CAD build for the part. Positions are in the model's coordinates, mm. A direction names the side the tool comes from. Round coordinates to 2 decimals unless told otherwise and drop trailing zeros. Loops run counter-clockwise (first coordinate to the right, second up) from the corner with the lowest first, then second, coordinate; pieces in that order, holes last.
Autodesk Fusion 360 part; units mm, degrees
box "BoxPrimitive1" add length 111 width 43 height 5 placed x (0, 1, 0) y (-1, 0, 0) z (0, 0, 1) at (43.0003, 0, 0)
sketch "Sketch6" plane through (0, 0, 0) normal (0, 0, -1) x (1, 0, 0)
  line L0 (0.0003, -111) -> (43.0003, -111)
  line L1 (43.0003, -111) -> (43.0003, 0)
  line L2 (43.0003, 0) -> (0.0003, 0)
  line L3 (0.0003, 0) -> (0.0003, -111)
  line L4 (0.0003, -93) -> (18.0003, -111)
  line L5 (6.5003, -22.25) -> (41.5003, -22.25) construction
  line L6 (41.5003, -22.25) -> (41.5003, -88.75) construction
  line L7 (41.5003, -88.75) -> (6.5003, -88.75) construction
  line L8 (6.5003, -88.75) -> (6.5003, -22.25) construction
  line L9 (6.5003, -22.25) -> (41.5003, -88.75) construction
  line L10 (6.5003, -88.75) -> (41.5003, -22.25) construction
  circle A0 centre (8.2003, -23.95) radius 0.8
  line L11 (38.2503, -87.75) -> (9.7503, -87.75)
  line L12 (9.7503, -87.75) -> (9.7503, -23.25)
  line L13 (9.7503, -23.25) -> (38.2503, -23.25)
  line L14 (38.2503, -23.25) -> (38.2503, -87.75)
  line L15 (38.2503, -87.75) -> (9.7503, -23.25) construction
  line L16 (9.7503, -87.75) -> (38.2503, -23.25) construction
  line L17 (18.2503, -91) -> (38.2503, -91)
  line L18 (38.2503, -91) -> (38.2503, -103)
  line L19 (38.2503, -103) -> (18.2503, -103)
  line L20 (18.2503, -103) -> (18.2503, -91)
  circle A1 centre (2.5003, -2.5) radius 1.2
  circle A2 centre (40.5003, -2.5) radius 1.2
  circle A3 centre (40.5003, -108.5) radius 1.2
  circle A4 centre (2.5003, -90.5) radius 1.2
  line L21 (24.0003, -111) -> (24.0003, 0) construction
  line L22 (0.0003, -55.5) -> (43.0003, -55.5) construction
  circle A5 centre (8.2003, -87.05) radius 0.8
  circle A6 centre (39.8003, -23.95) radius 0.8
  circle A7 centre (39.8003, -87.05) radius 0.8
  line L23 (18.2503, -91) -> (38.2503, -103) construction
  line L24 (38.2503, -91) -> (18.2503, -103) construction
  point P0 (24.0003, -55.5)
  point P1 (24.0003, -55.5)
  point P2 (24.0003, -55.5)
  point P3 (24.0003, -55.5)
  point P4 (28.2503, -97)
  dimension "d7" = 45
  dimension "d8" = 35
  dimension "d9" = 66.5
  dimension "d11" = 1.6
  dimension "d12" = 1.7
  dimension "d13" = 1.7
  dimension "d14" = 28.5
  dimension "d15" = 64.5
  dimension "d17" = 2.4
  dimension "d18" = 2.5
  dimension "d19" = 2.5
  dimension "d21" = 2.4
  dimension "d22" = 2.5
  dimension "d23" = 2.5
  dimension "d24" = 2.4
  dimension "d25" = 2.5
  dimension "d26" = 2.5
  dimension "d38" = 93
  dimension "d39" = 4.75
  dimension "d42" = 20
  dimension "d43" = 12
  dimension "d47" = 55.5
  dimension "d48" = 19
  dimension "d51" = 2.5
  dimension "d52" = 2.5
  dimension "d53" = 2.4
  dimension "d56" = 3.25
extrude "Extrude1" cut sketch "Sketch6" against normal through all contours L0 L3 L4 | L11 L12 L13 L14 | L17 L18 L19 L20 | A1 | A2 | A3 | A4
extrude "Extrude4" cut sketch "Sketch6" against normal blind 4 contours A0 | A5 | A6 | A7
thread "Thread2" thread offset 0 thread length 10
sketch "Sketch9" plane through (0, 0, 5) normal (0, 0, 1) x (-1, 0, 0)
  line L0 (-18.0003, -111) -> (-0.0003, -93)
  line L1 (-0.0003, -93) -> (-0.0003, 0)
  line L2 (-0.0003, 0) -> (-43.0003, 0)
  line L3 (-43.0003, 0) -> (-43.0003, -111)
  line L4 (-43.0003, -111) -> (-18.0003, -111)
  circle A0 centre (-40.5003, -108.5) radius 1.2
  line L5 (-18.2503, -91) -> (-18.2503, -103)
  line L6 (-18.2503, -103) -> (-38.2503, -103)
  line L7 (-38.2503, -103) -> (-38.2503, -91)
  line L8 (-38.2503, -91) -> (-18.2503, -91)
  circle A1 centre (-2.5003, -90.5) radius 1.2
  circle A2 centre (-40.5003, -2.5) radius 1.2
  line L9 (-38.2503, -87.75) -> (-38.2503, -23.25)
  line L10 (-38.2503, -23.25) -> (-9.7503, -23.25)
  line L11 (-9.7503, -23.25) -> (-9.7503, -87.75)
  line L12 (-9.7503, -87.75) -> (-38.2503, -87.75)
  circle A3 centre (-2.5003, -2.5) radius 1.2
  circle A4 centre (-2.5003, -2.5) radius 2
  circle A5 centre (-40.5003, -2.5) radius 2
  circle A6 centre (-2.5003, -90.5) radius 2
  circle A7 centre (-40.5003, -108.5) radius 2
  dimension "d32" = 4
  dimension "d33" = 4
  dimension "d34" = 4
  dimension "d35" = 4
extrude "Extrude3" cut sketch "Sketch9" against normal blind 2.5 contours A4 | A5 | A6 | A7
sketch "Sketch10" plane through (0, 0, 5) normal (0, 0, 1) x (-1, 0, 0)
  line L0 (-38.2503, -87.75) -> (-38.2503, -23.25)
  line L1 (-38.2503, -23.25) -> (-9.7503, -23.25)
  line L2 (-9.7503, -23.25) -> (-9.7503, -87.75)
  line L3 (-9.7503, -87.75) -> (-38.2503, -87.75)
  line L4 (-18.2503, -91) -> (-18.2503, -103)
  line L5 (-18.2503, -103) -> (-38.2503, -103)
  line L6 (-38.2503, -103) -> (-38.2503, -91)
  line L7 (-38.2503, -91) -> (-18.2503, -91)
  line L8 (-18.0003, -111) -> (-0.0003, -93)
  line L9 (-0.0003, -93) -> (-0.0003, 0)
  line L10 (-0.0003, 0) -> (-43.0003, 0)
  line L11 (-43.0003, 0) -> (-43.0003, -111)
  line L12 (-43.0003, -111) -> (-18.0003, -111)
  circle A0 centre (-40.5003, -108.5) radius 2
  circle A1 centre (-2.5003, -2.5) radius 2
  circle A2 centre (-2.5003, -90.5) radius 2
  circle A3 centre (-40.5003, -2.5) radius 2
fillet "Fillet1" radius 2 4 edges at (38.2503, 91, 2.5) (18.2503, 91, 2.5) (38.2503, 103, 2.5) (18.2503, 103, 2.5)
Item 1: Wall check: L1, parallel to Y at x = 28.5, z = 2; L2, parallel to X at y = 23.95, z = 1.25; L3, parallel to X at y = 87.5, z = 4.2. Give the ranges that are in metal, low to high.
Verdict:
L1: y = 0 to 23.25, 87.75 to 91, 103 to 111
L2: x = 0 to 7.4, 9 to 9.75, 38.25 to 39, 40.6 to 43
L3: x = 0 to 9.75, 38.25 to 43
Item 2: Cut at A-A (x = 24.5). List the corners of the cut face in (y, z), plus the area to 4 significant figures.
Verdict:
outline: (0, 0) - (23.25, 0) - (23.25, 5) - (0, 5) - close; (87.75, 0) - (91, 0) - (91, 5) - (87.75, 5) - close; (103, 0) - (111, 0) - (111, 5) - (103, 5) - close
area: 172.5 mm2
Item 3: Mould opens along Y. For faces 1 (the flat face through (22, 0, 2)), 2 (the cylindrical face through (18.82, 91.6, 2.54)), 3 (the cylindrical face through (18.85, 102.43, 2.54)), 4 (the flat face through (9, 102, 2)) say: released by +Y, released by -Y, zero draft, split by the parting line, or undercut.
Verdict:
face 1: released by -Y
face 2: undercut
face 3: undercut
face 4: released by +Y
Item 4: Cut at D-D (x = 15). List the corners of the cut face in (y, z), plus the area to 3 significant figures.
Verdict:
outline: (0, 0) - (23.25, 0) - (23.25, 5) - (0, 5) - close; (87.75, 0) - (108, 0) - (108, 5) - (87.75, 5) - close
area: 217 mm2
Item 5: Flat gauge pins, fed straight in: P1, Ø2.5, axis at y = 98.5, z = 2, coming from the -X side; P2, Ø1.4, axis at x = 39.8, y = 23.95, coming from the -Z side. Where does each tip first touch, or does it go through?
Verdict:
P1: stops at x = 4.25
P2: stops at z = 4
Item 6: Cut at B-B (y = 2.5). List the corners of the cut face in (x, z).
Verdict:
outline: (0, 0) - (1.3, 0) - (1.3, 2.5) - (0.5, 2.5) - (0.5, 5) - (0, 5) - close; (3.7, 0) - (39.3, 0) - (39.3, 2.5) - (38.5, 2.5) - (38.5, 5) - (4.5, 5) - (4.5, 2.5) - (3.7, 2.5) - close; (41.7, 0) - (43, 0) - (43, 5) - (42.5, 5) - (42.5, 2.5) - (41.7, 2.5) - close
Item 7: 3-axis set-ups, long thin cutter, end or side, ignore diameter. For faces 5 (the flat face through (39, 108, 2.5)), 6 (the flat face through (24, 87.75, 2)), 7 (the flat face through (0, 47, 2)): which of +Z, -Z, +X, -X, +Y, -Y reach the whole face in a straight line?
Verdict:
face 5: +Z
face 6: +Z, -Z
face 7: +Z, -Z, -X, +Y, -Y
Item 8: Cut at C-C (y = 26). List the corners of the cut face in (x, z), plus the area to 3 significant figures.
Verdict:
outline: (0, 0) - (9.75, 0) - (9.75, 5) - (0, 5) - close; (38.25, 0) - (43, 0) - (43, 5) - (38.25, 5) - close
area: 72.5 mm2
